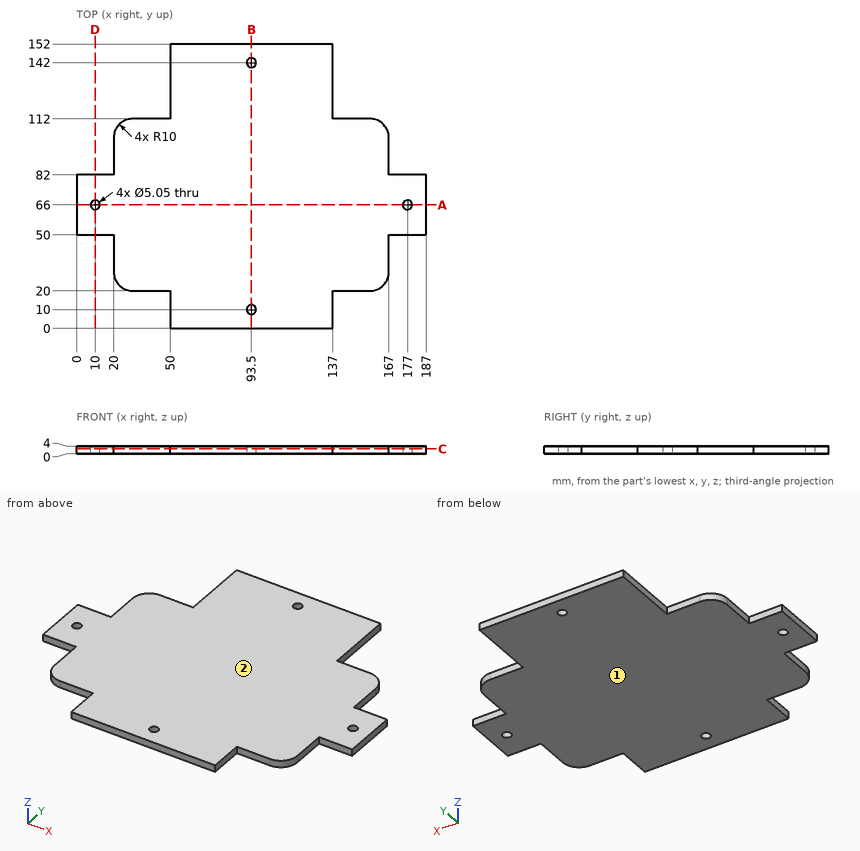
Part print with two shaded views. Sizes in mm from the minimum x, y, z corner. Give positions to 0.01 mm unless a question says otherwise; leave off trailing zeros. Order: outer loops, then holes, each group sorted by start corner. A loop starts at its lowest first (then second) coordinate and runs counter-clockwise, first axis right, second up. Notation, with made-up numbers: M 8,-28.75 L 26,-28.75 A10 cw 26,-14.75 Z; hole C 51.25,-37 d11. An arc over 180 degrees is marked long. Write item = value, one per line.
Q1. Cut at B-B, the plane x = 93.5. List the corners of the cut face in (y, z) (3 decimals), then the cut area to 3 significant figures.
Derived:
outline = M 0,0 L 7.475,0 L 7.475,4 L 0,4 Z; M 12.525,0 L 139.475,0 L 139.475,4 L 12.525,4 Z; M 144.525,0 L 152,0 L 152,4 L 144.525,4 Z
area = 568 mm2
Q2. Cut at C-C, the plane z = 2.65. List the corners of the cut face in (x, y) (3 decimals), then the cut area to 3 significant figures.
Derived:
outline = M 0,50 L 20,50 L 20,30 A10 ccw 30,20 L 50,20 L 50,0 L 137,0 L 137,20 L 157,20 A10 ccw 167,30 L 167,50 L 187,50 L 187,82 L 167,82 L 167,102 A10 ccw 157,112 L 137,112 L 137,152 L 50,152 L 50,112 L 30,112 A10 ccw 20,102 L 20,82 L 0,82 Z; hole C 10,66 d5.05; hole C 93.5,10 d5.05; hole C 93.5,142 d5.05; hole C 177,66 d5.05
area = 19,900 mm2
Q3. Cut at D-D, the plane x = 10. List the corners of the cut face in (y, z) (3 decimals), then the cut area to 3 significant figures.
Derived:
outline = M 50,0 L 63.475,0 L 63.475,4 L 50,4 Z; M 68.525,0 L 82,0 L 82,4 L 68.525,4 Z
area = 108 mm2
Q4. Cut at A-A, the plane y = 66. List the corners of the cut face in (x, z) (3 decimals).
Derived:
outline = M 0,0 L 7.475,0 L 7.475,4 L 0,4 Z; M 12.525,0 L 174.475,0 L 174.475,4 L 12.525,4 Z; M 179.525,0 L 187,0 L 187,4 L 179.525,4 Z
Q5. Flat gauge pins, fed straight in: pin 1 (1.2 mm diameter, centred on y = 13.5, z = 1.5, fed in from -X); pin 2 (2 mm diameter, centred on y = 136, z = 3, fed in from +X); pin 3 (1.2 mm diameter, centred on y = 87, z = 1.5, fed in from +X). Where does each tip first touch, or does it go through?
Derived:
pin_1 = 50
pin_2 = 137
pin_3 = 167
Q6. Two-plate mould, pull along Z, no slides. Class the marked faces 1 and 2: pulls with the +Z half, pulls with the -Z half, needs draft (parallel to the pull), parting line crosses it, or undercut.
Derived:
face_1 = pulls with the -Z half
face_2 = pulls with the +Z half
Q7. Drill centre lines: line 1 (Y direction, x = 10, z = 2.9) (3 decimals); line 2 (Y direction, x = 93.5, z = 2.7) (3 decimals); line 3 (X direction, y = 142, z = 1.2) (3 decimals). Where is each one in solid material? Low to high. Write a range as [from, to].
Derived:
line_1 = [50, 63.475], [68.525, 82]
line_2 = [0, 7.475], [12.525, 139.475], [144.525, 152]
line_3 = [50, 90.975], [96.025, 137]
